```python
from build123d import *

# Parameters (mm, degrees)
SKETCH1_W                    = 300
SKETCH1_H                    = 820
BOSS_EXTRUDE1_DEPTH          = 2
CONVERT_SOLID1_OUTLINE_W     = 300
CONVERT_SOLID1_OUTLINE_H     = 820
CONVERT_SOLID1_DEPTH         = 0.5
EDGE_FLANGE1_STRIP_W         = 10
EDGE_FLANGE1_STRIP_H         = 1.5
EDGE_FLANGE1_STRIP_CUT_DEPTH = 820
EDGE_FLANGE1_DEPTH           = 820
EDGE_FLANGE2_STRIP_W         = 10
EDGE_FLANGE2_STRIP_H         = 1.5
EDGE_FLANGE2_STRIP_CUT_DEPTH = 820
EDGE_FLANGE2_DEPTH           = 820
CUT_EXTRUDE1_DEPTH           = 1226.561095988


# Read off the part's stored shape, not the designer's step: Convert-Solid1
# Sheet-metal steps are written as plain solids
with BuildPart() as part:
    # Sketch1 → Boss-Extrude1 (new body)
    with BuildSketch(Plane.XY):
        with Locations((150, 410)):
            Rectangle(SKETCH1_W, SKETCH1_H)
    extrude(amount=BOSS_EXTRUDE1_DEPTH)

    # Convert-Solid1 outline → Convert-Solid1 (cut)
    with BuildSketch(Plane.XY):
        with Locations((150, 410)):
            Rectangle(CONVERT_SOLID1_OUTLINE_W, CONVERT_SOLID1_OUTLINE_H)
    extrude(amount=CONVERT_SOLID1_DEPTH, mode=Mode.SUBTRACT)

    # Edge-Flange1 strip (across the edge) → Edge-Flange1 strip cut (cut)
    with BuildSketch(Plane(origin=(300, 820, 0.5), x_dir=(-1, 0, 0), z_dir=(0, -1, 0))):
        with Locations((-3, -0.75)):
            Rectangle(EDGE_FLANGE1_STRIP_W, EDGE_FLANGE1_STRIP_H)
    extrude(amount=EDGE_FLANGE1_STRIP_CUT_DEPTH, mode=Mode.SUBTRACT)

    # Edge-Flange1 section (across the edge) → Edge-Flange1 (add)
    with BuildSketch(Plane(origin=(300, 820, 0.5), x_dir=(-1, 0, 0), z_dir=(0, -1, 0))):
        with BuildLine():
            Line((-1.5, 2), (-1.5, 138.5))
            Line((-1.5, 138.5), (0, 138.5))
            Line((0, 138.5), (0, 2))
            ThreePointArc((0, 2), (0.585786438, 0.585786438), (2, 0))
            Line((2, 0), (2, -1.5))
            ThreePointArc((2, -1.5), (-0.474873734, -0.474873734), (-1.5, 2))
        make_face()
    extrude(amount=EDGE_FLANGE1_DEPTH)

    # Edge-Flange2 strip (across the edge) → Edge-Flange2 strip cut (cut)
    with BuildSketch(Plane(origin=(301.5, 0, -138), x_dir=(0, 0, 1), z_dir=(0, 1, 0))):
        with Locations((-3, -0.75)):
            Rectangle(EDGE_FLANGE2_STRIP_W, EDGE_FLANGE2_STRIP_H)
    extrude(amount=EDGE_FLANGE2_STRIP_CUT_DEPTH, mode=Mode.SUBTRACT)

    # Edge-Flange2 section (across the edge) → Edge-Flange2 (add)
    with BuildSketch(Plane(origin=(301.5, 0, -138), x_dir=(0, 0, 1), z_dir=(0, 1, 0))):
        with BuildLine():
            Line((-1.5, 2), (-1.5, 598.5))
            Line((-1.5, 598.5), (0, 598.5))
            Line((0, 598.5), (0, 2))
            ThreePointArc((0, 2), (0.585786438, 0.585786438), (2, 0))
            Line((2, 0), (2, -1.5))
            ThreePointArc((2, -1.5), (-0.474873734, -0.474873734), (-1.5, 2))
        make_face()
    extrude(amount=EDGE_FLANGE2_DEPTH)

    # Sketch12 → Cut-Extrude1 (cut, through all)
    with BuildSketch(Plane.XY.offset(-138)):
        with BuildLine():
            Line((395.117398745, 789.936561894), (475.117398745, 789.936561894))
            ThreePointArc((475.117398745, 789.936561894), (482.188466557, 787.007629706), (485.117398745, 779.936561894))
            Line((485.117398745, 779.936561894), (485.117398745, 749.936561894))
            ThreePointArc((485.117398745, 749.936561894), (482.188466557, 742.865494082), (475.117398745, 739.936561894))
            Line((475.117398745, 739.936561894), (395.117398745, 739.936561894))
            ThreePointArc((395.117398745, 739.936561894), (388.046330933, 742.865494082), (385.117398745, 749.936561894))
            Line((385.117398745, 749.936561894), (385.117398745, 779.936561894))
            ThreePointArc((385.117398745, 779.936561894), (388.046330933, 787.007629706), (395.117398745, 789.936561894))
        make_face()
    extrude(amount=-CUT_EXTRUDE1_DEPTH, mode=Mode.SUBTRACT)


solid = part.part
```
Source: CAD feature listing. Evaluate the final solid. Frame: model axes, mm. A direction names the side the tool comes from. Coordinates: 2 decimals unless noted, no trailing zeros. Write each loop counter-clockwise with the first axis right and the second up, starting at its lowest first coordinate (ties: lowest second). Pieces come first, ordered by that corner, then holes. Notation, with made-up numbers: (15, 64) - (72, 64) arc R29 ccw to (72, 85) - close; hole circle Ø4 at (7, 49). An arc over 180 degrees is marked (long way). Answer as a JSON object with one key per item and string values.
Q1. First-contact query: pin 1 Ø12 at (x, y) = (739, 182) entering from +Z; pin 2 Ø5 at (y, z) = (599, -120.5) entering from -X; pin 3 Ø2 at (y, z) = (383.5, -107) entering from +X. Flat tips, straight axial feed; report the tip coordinate or a pass-through.
Ans:
{"pin 1": "stops at z = -138", "pin 2": "stops at x = 300", "pin 3": "stops at x = 301.5"}
Q2. Section query D-D, the plane x = 569.5. Output: boundary loops of the cut face in (y, z), plus the area to 3 significant figures.
Ans:
{"outline": "(0, -139.5) - (820, -139.5) - (820, -138) - (0, -138) - close", "area": "1,230 mm2"}
Q3. Section query C-C, the plane z = -53. Output: boundary loops of the cut face in (x, y), plus the area to 3 significant figures.
Ans:
{"outline": "(300, 0) - (301.5, 0) - (301.5, 820) - (300, 820) - close", "area": "1,230 mm2"}
Q4. Section query B-B, the plane y = 458. Output: boundary loops of the cut face in (x, z), plus the area to 3 significant figures.
Ans:
{"outline": "(0, 0.5) - (298, 0.5) arc R2 cw to (300, -1.5) - (300, -136) arc R3.5 ccw to (303.5, -139.5) - (900, -139.5) - (900, -138) - (303.5, -138) arc R2 cw to (301.5, -136) - (301.5, -1.5) arc R3.5 ccw to (298, 2) - (0, 2) - close", "area": "1,560 mm2"}
Q5. Material intervals for line 1 (X direction, y = 783, z = -111); line 2 (Z direction, x = 748, y = 574); line 3 (Z direction, x = 47, y = 441.5), sorted ascending. Write a range as [from, to].
Ans:
{"line 1": "x = [300, 301.5]", "line 2": "z = [-139.5, -138]", "line 3": "z = [0.5, 2]"}
Q6. Section query A-A, the plane x = 465. Output: boundary loops of the cut face in (y, z).
Ans:
{"outline": "(0, -139.5) - (739.94, -139.5) - (739.94, -138) - (0, -138) - close; (789.94, -139.5) - (820, -139.5) - (820, -138) - (789.94, -138) - close"}
Q7. Set-up query: faces 1 (the flat face through (147, 416, 0.5)), 2 (the flat face through (301.5, 416, -68)), 3 (the flat face through (598, 404, -139.5)). Return all of +Z, -Z, +X, -X, +Y, -Y with unobstructed straight access to the full face (end or side cutting, diameter ignored); none if empty.
Ans:
{"face 1": "-Z, -X, +Y, -Y", "face 2": "+Z, +X, +Y, -Y", "face 3": "-Z, +X, -X, +Y, -Y"}
